Here's the drawing with two shaded views (mm, measured from the low corner). I have some questions. Coordinates: 2 decimals unless noted, no trailing zeros. Loops run counter-clockwise (first coordinate to the right, second up) from the corner with the lowest first, then second, coordinate; pieces in that order, holes last.
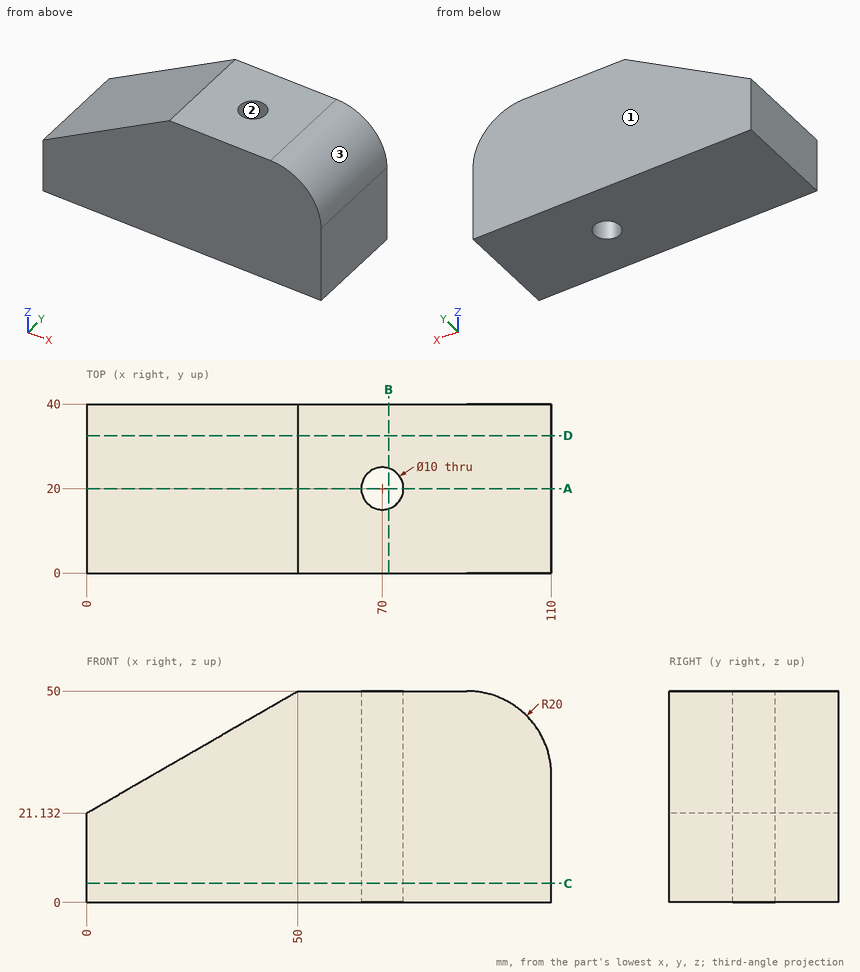
(1) I want a section at B-B on x = 71.5. Write out the boundary of the cut face in (y, z).
Check values:
outline: (0, 0) - (15.23, 0) - (15.23, 50) - (0, 50) - close; (24.77, 0) - (40, 0) - (40, 50) - (24.77, 50) - close
(2) If we mould it in two halves opening along Y, with no side actions, what happens to the marked faces 1, 2 and 3? For each: released by +Y, released by -Y, zero draft, split by the parting line, or undercut.
Check values:
face 1: released by +Y
face 2: undercut
face 3: zero draft
(3) I want a section at A-A on y = 20. Write out the boundary of the cut face in (x, z).
Check values:
outline: (0, 0) - (65, 0) - (65, 50) - (50, 50) - (0, 21.13) - close; (75, 0) - (110, 0) - (110, 30) arc R20 ccw to (90, 50) - (75, 50) - close
(4) I want a section at D-D on y = 32.5. Write out the boundary of the cut face in (x, z).
Check values:
outline: (0, 0) - (110, 0) - (110, 30) arc R20 ccw to (90, 50) - (50, 50) - (0, 21.13) - close
(5) I want a section at C-C on z = 4.5. Write out the boundary of the cut face in (x, y).
Check values:
outline: (0, 0) - (110, 0) - (110, 40) - (0, 40) - close; hole circle Ø10 at (70, 20)
(6) I'm going to push flat-ended pins straight in: pin 1 (8 mm diameter, centred on x = 70, y = 20, fed in from +Z); pin 2 (5 mm diameter, centred on x = 38.5, y = 11, fed in from +Z) (1 decimal). Where does each tip first touch, or does it pass through?
Check values:
pin 1: passes through
pin 2: stops at z = 44.8
(7) If I drill on probe 1 along Y at (x, z) = (70, 22.5); probe 2 along X at (y, z) = (20, 19.5); probe 3 along Y at (x, z) = (68, 41), over which ranges is the centre line in solid material (lowest first)?
Check values:
probe 1: y = 0 to 15, 25 to 40
probe 2: x = 0 to 65, 75 to 110
probe 3: y = 0 to 15.42, 24.58 to 40
